Source: CAD feature listing. Evaluate the final solid. Frame: model axes, mm. Face numbers are marked on the shaded views. A direction names the side the tool comes from. Give positions to 0.01 mm unless a question says otherwise; leave off trailing zeros. Loops run counter-clockwise (first coordinate to the right, second up) from the corner with the lowest first, then second, coordinate; pieces in that order, holes last. Notation, with made-up numbers: (0, 19.5) -> (28, 19.5) arc R8 ccw to (28, 26.5) -> close; hole circle Ø1 at (85.25, 43.25). An arc over 180 degrees is marked (long way). Return JSON: item names as keys, results as strings. Group by question number.
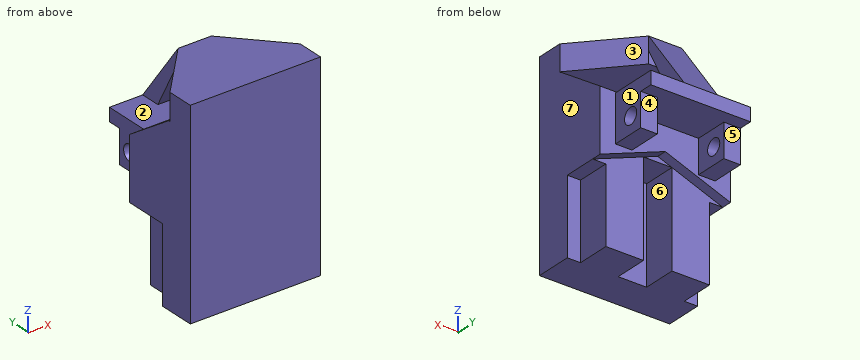
```python
from build123d import *

# Parameters (mm, degrees)
BOSS_EXTRUDE2_DEPTH      = 10
BOSS_EXTRUDE2_DEPTH_BACK = 10
SKETCH2_W                = 30
SKETCH2_H                = 12
SKETCH11_W               = 2.5
SKETCH11_H               = 5
BOSS_EXTRUDE5_DEPTH      = 5
SKETCH12_R               = 1.2
CUT_EXTRUDE3_DEPTH       = 5
SKETCH13_W               = 15
SKETCH13_H               = 2
BOSS_EXTRUDE6_DEPTH      = 7
SKETCH16_W               = 30
SKETCH16_H               = 12
CUT_EXTRUDE4_DEPTH       = 0.2
CUT_EXTRUDE5_DEPTH       = 1.5
CUT_EXTRUDE6_DEPTH       = 31
SKETCH23_W               = 4.283577098
SKETCH23_H               = 14.196829294
CUT_EXTRUDE7_DEPTH       = 5
SKETCH24_W               = 2
SKETCH24_H               = 11.325
CUT_EXTRUDE8_DEPTH       = 5
CUT_EXTRUDE9_DEPTH       = 4


with BuildPart() as part:
    # Sketch2 → Boss-Extrude2 (new, two sides: drawn at the far end of the back side and taken through both)
    with BuildSketch(Plane(origin=(0, 0, 0), x_dir=(0, 0, -1), z_dir=(1, 0, 0)).offset(-BOSS_EXTRUDE2_DEPTH_BACK)):
        with Locations((15, 6)):
            Rectangle(SKETCH2_W, SKETCH2_H)
    extrude(amount=BOSS_EXTRUDE2_DEPTH + BOSS_EXTRUDE2_DEPTH_BACK)

    # Sketch11 → Boss-Extrude5 (add)
    with BuildSketch(Plane(origin=(0, 12, 0), x_dir=(1, 0, 0), z_dir=(0, 1, 0))):
        with Locations((-6.25, 14)):
            Rectangle(SKETCH11_W, SKETCH11_H)
    boss_extrude5 = extrude(amount=BOSS_EXTRUDE5_DEPTH)

    # Sketch12 → Cut-Extrude3 (cut)
    with BuildSketch(Plane(origin=(-5, 0, 0), x_dir=(0, 0, -1), z_dir=(1, 0, 0))):
        with Locations((14, 15)):
            Circle(SKETCH12_R)
    cut_extrude3 = extrude(amount=-CUT_EXTRUDE3_DEPTH, mode=Mode.SUBTRACT)

    # Mirror2: Boss-Extrude5, Cut-Extrude3 across plane
    add(boss_extrude5.mirror(Plane.ZY))
    add(cut_extrude3.mirror(Plane.ZY), mode=Mode.SUBTRACT)

    # Sketch13 → Boss-Extrude6 (add)
    with BuildSketch(Plane(origin=(0, 12, 0), x_dir=(1, 0, 0), z_dir=(0, 1, 0))):
        with Locations((0, 10.5)):
            Rectangle(SKETCH13_W, SKETCH13_H)
    extrude(amount=BOSS_EXTRUDE6_DEPTH)

    # Sketch16 → Cut-Extrude4 (cut)
    with BuildSketch(Plane(origin=(10, 0, 0), x_dir=(0, 0, -1), z_dir=(1, 0, 0))):
        with Locations((15, 6)):
            Rectangle(SKETCH16_W, SKETCH16_H)
    cut_extrude4 = extrude(amount=-CUT_EXTRUDE4_DEPTH, mode=Mode.SUBTRACT)

    # Mirror3: Cut-Extrude4 across plane
    add(cut_extrude4.mirror(Plane.ZY), mode=Mode.SUBTRACT)

    # Sketch5 → Cut-Extrude5 (cut)
    with BuildSketch(Plane(origin=(0, 12, 0), x_dir=(1, 0, 0), z_dir=(0, 1, 0))):
        Polygon((-10, 18.75), (-10, 30), (10, 30), (10, 18.75), (0, 15), align=None)
    extrude(amount=-CUT_EXTRUDE5_DEPTH, mode=Mode.SUBTRACT)

    # Sketch20 → Loft1 section 0
    with BuildSketch(Plane(origin=(0, 12, 0), x_dir=(1, 0, 0), z_dir=(0, 1, 0))):
        with BuildLine():
            Line((-2.5, 2), (2.5, 2))
            Line((2.5, 2), (2.5, 0))
            Line((2.5, 0), (-2.5, 0))
            Line((-2.5, 0), (-2.5, 2))
        make_face()
    # Sketch19 → Loft1 section 1
    with BuildSketch(Plane.XY.offset(-9.5)):
        with BuildLine():
            Line((2.5, 16), (-2.5, 16))
            Line((-2.5, 16), (-2.5, 19))
            Line((-2.5, 19), (2.5, 19))
            Line((2.5, 19), (2.5, 16))
        make_face()
    loft()

    # Sketch22 → Cut-Extrude6 (cut)
    with BuildSketch(Plane.ZY.offset(9.8)):
        Polygon((-9.3375, 12), (-3.836516703, 4.014793252), (-3.836516703, 12), align=None)
    extrude(amount=-CUT_EXTRUDE6_DEPTH, mode=Mode.SUBTRACT)

    # Sketch23 → Cut-Extrude7 (cut)
    with BuildSketch(Plane(origin=(0, 10.5, 0), x_dir=(1, 0, 0), z_dir=(0, 1, 0))):
        with Locations((0, 22.901585353)):
            Rectangle(SKETCH23_W, SKETCH23_H)
    extrude(amount=-CUT_EXTRUDE7_DEPTH, mode=Mode.SUBTRACT)

    # Sketch24 → Cut-Extrude8 (cut)
    with BuildSketch(Plane(origin=(0, 10.5, 0), x_dir=(1, 0, 0), z_dir=(0, 1, 0))):
        with Locations((8.8, 24.3375)):
            Rectangle(SKETCH24_W, SKETCH24_H)
    cut_extrude8 = extrude(amount=-CUT_EXTRUDE8_DEPTH, mode=Mode.SUBTRACT)

    # Mirror4: Cut-Extrude8 across plane
    add(cut_extrude8.mirror(Plane.ZY), mode=Mode.SUBTRACT)

    # Sketch25 → Cut-Extrude9 (cut)
    with BuildSketch(Plane.XY):
        Polygon((-9.8, 12), (-9.8, 4.014793252), (-2.5, 12), align=None)
    cut_extrude9 = extrude(amount=-CUT_EXTRUDE9_DEPTH, mode=Mode.SUBTRACT)

    # Mirror5: Cut-Extrude9 across plane
    add(cut_extrude9.mirror(Plane.ZY), mode=Mode.SUBTRACT)


solid = part.part
```
1) Contact query for flat-ended pins moving along their axis: P1, Ø4.5, axis at x = 0, z = -23.5, coming from the +Y side; P2, Ø3, axis at y = 10.5, z = -24.5, coming from the -X side; P3, Ø1, axis at x = -0.5, y = 15.5, coming from the +Z side. Output: stop coordinate, or through.
2) Cut plane C-C on x = 6.5. Return loops of the section in (y, z).
3) Material intervals for line 1 (X direction, y = 16.75, z = -15); line 2 (Y direction, x = -5.8, z = -14); line 3 (X direction, y = 7, z = -18.5), sorted ascending.
4) Cut plane A-A on z = -14. Return loops of the section in (x, y).
5) Mould query, pull axis X, two halves, no side actions, for the marked faces 5, 6 and 7. Classes: released by +X, released by -X, zero draft, split by the parting line, or undercut.
6) Cut plane B-B on z = -21.5. Return loops of the section in (x, y).
7) Cut plane D-D on y = 15. Count the separate pieces of the cut face and the enclosed holes in it, then the cut area to 3 significant figures.
8) Reachability of the marked faces 1, 2, 3 and 4 from +Z, -Z, +X, -X, +Y, -Y: full face, straight path, thin tool, end or side. Return the list, or none.
Calculated:
{
 "1": {"P1": "y = 10.5", "P2": "x = -7.8", "P3": "z = -4.07"},
 "2": {"outline": "(0, -30) -> (10.5, -30) -> (10.5, -17.44) -> (12, -17.44) -> (12, -16.5) -> (17, -16.5) -> (17, -11.5) -> (19, -11.5) -> (19, -9.5) -> (12, -9.5) -> (12, -9.34) -> (4.01, -3.84) -> (7.62, -3.84) -> (7.62, 0) -> (0, 0) -> close; hole circle Ø2.4 at (15, -14)"},
 "3": {"line 1": "-7.5 to -5, 5 to 7.5", "line 2": "0 to 13.8, 16.2 to 17", "line 3": "-9.8 to -2.14, 2.14 to 9.8"},
 "4": {"outline": "(-9.8, 0) -> (9.8, 0) -> (9.8, 12) -> (7.5, 12) -> (7.5, 13.8) -> (5, 13.8) -> (5, 12) -> (-5, 12) -> (-5, 13.8) -> (-7.5, 13.8) -> (-7.5, 12) -> (-9.8, 12) -> close; (-7.5, 16.2) -> (-5, 16.2) -> (-5, 17) -> (-7.5, 17) -> close; (5, 16.2) -> (7.5, 16.2) -> (7.5, 17) -> (5, 17) -> close"},
 "5": {"face 5": "zero draft", "face 6": "undercut", "face 7": "released by +X"},
 "6": {"outline": "(-9.8, 0) -> (9.8, 0) -> (9.8, 5.5) -> (7.8, 5.5) -> (7.8, 10.5) -> (2.14, 10.5) -> (2.14, 5.5) -> (-2.14, 5.5) -> (-2.14, 10.5) -> (-7.8, 10.5) -> (-7.8, 5.5) -> (-9.8, 5.5) -> close"},
 "7": {"separate pieces": "4", "enclosed holes": "0", "area": "60.8 mm2"},
 "8": {"face 1": "+Z, -Z, +X, +Y", "face 2": "none", "face 3": "+Z, +X, +Y", "face 4": "-Z, +X, -X, +Y"}
}
